from build123d import *

# Parameters (mm, degrees)
ESQUISSE1_W             = 40
ESQUISSE1_H             = 35
ESQUISSE1_W_2           = 36
ESQUISSE1_H_2           = 31
BOSS_EXTRU_1_DEPTH      = 5.5
ESQUISSE2_W             = 40
ESQUISSE2_H             = 35
BOSS_EXTRU_2_DEPTH      = 2
ENL_V_MAT_EXTRU_1_REACH = 42
BOSS_EXTRU_3_DEPTH      = 7
ENL_V_MAT_EXTRU_2_REACH = 11
ESQUISSE9_W             = 7.5
ESQUISSE9_H             = 12
D_GAGEMENT_M31_D        = 3.4
CONG_1_R                = 2.5
BOSS_EXTRU_6_DEPTH      = 1.5


with BuildPart() as part:
    # Esquisse1 → Boss.-Extru.1 (new body)
    with BuildSketch(Plane.XY):
        with Locations((16.877269095, -24.858015503)):
            Rectangle(ESQUISSE1_W, ESQUISSE1_H)
        with Locations((16.877269095, -24.858015503)):
            Rectangle(ESQUISSE1_W_2, ESQUISSE1_H_2, mode=Mode.SUBTRACT)
    extrude(amount=BOSS_EXTRU_1_DEPTH)

    # Esquisse2 → Boss.-Extru.2 (add)
    with BuildSketch(Plane.XY.offset(5.5)):
        with Locations((16.877269095, -24.858015503)):
            Rectangle(ESQUISSE2_W, ESQUISSE2_H)
    extrude(amount=BOSS_EXTRU_2_DEPTH)

    # Esquisse3 → Enlèv. mat.-Extru.1 (cut, up to next)
    with BuildSketch(Plane(origin=(36.877269095, 0, 0), x_dir=(0, 0, -1), z_dir=(1, 0, 0)), mode=Mode.PRIVATE) as enl_v_mat_extru_1_sk1:
        with BuildLine():
            Line((0, -22.358015503), (0, -27.358015503))
            ThreePointArc((0, -27.358015503), (-2.5, -24.858015503), (0, -22.358015503))
        make_face()
    enl_v_mat_extru_1_tool1 = extrude(enl_v_mat_extru_1_sk1.sketch, amount=-ENL_V_MAT_EXTRU_1_REACH, mode=Mode.PRIVATE) & part.part
    add(enl_v_mat_extru_1_tool1.solids().sort_by_distance((36.877269, -24.858016, 1.061033))[0], mode=Mode.SUBTRACT)

    # Esquisse4 → Boss.-Extru.3 (add)
    with BuildSketch(Plane(origin=(0, 0, 5.5), x_dir=(-1, 0, 0), z_dir=(0, 0, -1))):
        with BuildLine():
            ThreePointArc((-34.877269095, -13.919753195), (-30.579172056, -13.656112542), (-30.315531404, -9.358015503))
            Line((-30.315531404, -9.358015503), (-34.877269095, -9.358015503))
            Line((-34.877269095, -9.358015503), (-34.877269095, -13.919753195))
        make_face()
        with BuildLine():
            Line((-34.877269095, -32.858015503), (-17.877269095, -32.858015503))
            Line((-17.877269095, -32.858015503), (-17.877269095, -40.358015503))
            Line((-17.877269095, -40.358015503), (-15.877269095, -40.358015503))
            Line((-15.877269095, -40.358015503), (-15.877269095, -31.858015503))
            ThreePointArc((-15.877269095, -31.858015503), (-16.170162314, -31.150908722), (-16.877269095, -30.858015503))
            Line((-16.877269095, -30.858015503), (-34.877269095, -30.858015503))
            Line((-34.877269095, -30.858015503), (-34.877269095, -32.858015503))
        make_face()
        with BuildLine():
            Line((-34.877269095, -35.796277812), (-34.877269095, -40.358015503))
            Line((-34.877269095, -40.358015503), (-30.315531404, -40.358015503))
            ThreePointArc((-30.315531404, -40.358015503), (-30.579172056, -36.059918465), (-34.877269095, -35.796277812))
        make_face()
        with BuildLine():
            Line((-17.877269095, -16.858015503), (-34.877269095, -16.858015503))
            Line((-34.877269095, -16.858015503), (-34.877269095, -18.858015503))
            Line((-34.877269095, -18.858015503), (-16.877269095, -18.858015503))
            ThreePointArc((-16.877269095, -18.858015503), (-16.170162314, -18.565122285), (-15.877269095, -17.858015503))
            Line((-15.877269095, -17.858015503), (-15.877269095, -9.358015503))
            Line((-15.877269095, -9.358015503), (-17.877269095, -9.358015503))
            Line((-17.877269095, -9.358015503), (-17.877269095, -16.858015503))
        make_face()
        with BuildLine():
            Line((-3.439006787, -40.358015503), (1.122730905, -40.358015503))
            Line((1.122730905, -40.358015503), (1.122730905, -35.796277812))
            ThreePointArc((1.122730905, -35.796277812), (-3.175366134, -36.059918465), (-3.439006787, -40.358015503))
        make_face()
        with BuildLine():
            Line((1.122730905, -13.919753195), (1.122730905, -9.358015503))
            Line((1.122730905, -9.358015503), (-3.439006787, -9.358015503))
            ThreePointArc((-3.439006787, -9.358015503), (-3.175366134, -13.656112542), (1.122730905, -13.919753195))
        make_face()
    extrude(amount=BOSS_EXTRU_3_DEPTH)

    # Esquisse9 → Enlèv. mat.-Extru.2 (cut, up to next)
    with BuildSketch(Plane(origin=(6.5, 0, 7.5), x_dir=(-1, 0, 0), z_dir=(0, 0, -1)), mode=Mode.PRIVATE) as enl_v_mat_extru_2_sk1:
        with Locations((-0.377269095, -24.858015503)):
            Rectangle(ESQUISSE9_W, ESQUISSE9_H)
    enl_v_mat_extru_2_tool1 = extrude(enl_v_mat_extru_2_sk1.sketch, amount=ENL_V_MAT_EXTRU_2_REACH, mode=Mode.PRIVATE) & part.part
    add(enl_v_mat_extru_2_tool1.solids().sort_by_distance((6.877269, -24.858016, 7.5))[0], mode=Mode.SUBTRACT)

    # Dégagement M31 (through all)
    with Locations(Plane.XY.offset(7.5)):
        with Locations((0.877269095, -11.358015503), (32.877269095, -38.358015503), (32.877269095, -11.358015503), (0.877269095, -38.358015503)):
            Hole(D_GAGEMENT_M31_D / 2)

    # Congé1
    cong_1_edges = [part.edges().sort_by_distance(p)[0] for p in [
        (-3.122730905, -7.358015503, 3.75),
        (36.877269095, -7.358015503, 3.75),
        (36.877269095, -42.358015503, 3.75),
        (-3.122730905, -42.358015503, 3.75),
    ]]
    fillet(cong_1_edges, radius=CONG_1_R)

    # Esquisse13 → Boss.-Extru.6 (add)
    with BuildSketch(Plane(origin=(0, 0, 0), x_dir=(-1, 0, 0), z_dir=(0, 0, -1))):
        with BuildLine():
            Line((-35.877269095, -27.358015503), (-34.877269095, -27.358015503))
            Line((-34.877269095, -27.358015503), (-34.877269095, -39.858015503))
            ThreePointArc((-34.877269095, -39.858015503), (-34.730822486, -40.211568894), (-34.377269095, -40.358015503))
            Line((-34.377269095, -40.358015503), (0.622730905, -40.358015503))
            ThreePointArc((0.622730905, -40.358015503), (0.976284295, -40.211568894), (1.122730905, -39.858015503))
            Line((1.122730905, -39.858015503), (1.122730905, -9.861767147))
            ThreePointArc((1.122730905, -9.861767147), (0.975185464, -9.505560944), (0.618979261, -9.358015503))
            Line((0.618979261, -9.358015503), (-34.377269095, -9.358015503))
            ThreePointArc((-34.377269095, -9.358015503), (-34.730822486, -9.504462113), (-34.877269095, -9.858015503))
            Line((-34.877269095, -9.858015503), (-34.877269095, -22.358015503))
            Line((-34.877269095, -22.358015503), (-35.877269095, -22.358015503))
            Line((-35.877269095, -22.358015503), (-35.877269095, -9.858015503))
            ThreePointArc((-35.877269095, -9.858015503), (-35.437929267, -8.797355332), (-34.377269095, -8.358015503))
            Line((-34.377269095, -8.358015503), (0.622730905, -8.358015503))
            ThreePointArc((0.622730905, -8.358015503), (1.683391077, -8.797355332), (2.122730905, -9.858015503))
            Line((2.122730905, -9.858015503), (2.122730905, -39.858015503))
            ThreePointArc((2.122730905, -39.858015503), (1.683391077, -40.918675675), (0.622730905, -41.358015503))
            Line((0.622730905, -41.358015503), (-34.377269095, -41.358015503))
            ThreePointArc((-34.377269095, -41.358015503), (-35.437929267, -40.918675675), (-35.877269095, -39.858015503))
            Line((-35.877269095, -39.858015503), (-35.877269095, -27.358015503))
        make_face()
    extrude(amount=BOSS_EXTRU_6_DEPTH)


solid = part.part
For this review, take the finished solid that the model builds, in its own axes (mm). A direction names the side the tool comes from. Give positions to 0.01 mm unless a question says otherwise; leave off trailing zeros. Loops run counter-clockwise (first coordinate to the right, second up) from the corner with the lowest first, then second, coordinate; pieces in that order, holes last. Notation, with made-up numbers: (2.5, 68) -> (45.5, 68) arc R15 cw to (45.5, 90) -> close; hole circle Ø8 at (-5, 2). An arc over 180 degrees is marked (long way). One line per question, with ' | ' between items.
1) For faces 1 (the flat face through (17, -8.358, -1)), 2 (the flat face through (7, -18.858, 7)), 3 (the flat face through (35.4, -27.358, -0.7)), 4 (the cylindrical face through (16.178, -18.573, 2.049)), list the 3-axis set-ups (+Z, -Z, +X, -X, +Y, -Y) from which the entire face can be reached by the end or side of a thin tool; tool diameter is ignored.
Resolved:
face 1: -Z, +X, -X, +Y | face 2: +Z, -Z | face 3: -Z, +X | face 4: -Z
2) To check wall thickness, follow probe 1 along Y at (x, z) = (22.5, 1.75); probe 2 along Y at (x, z) = (18, -1); probe 3 along X at (y, z) = (-18, 3). State the ranges of each line that lie inside material, in increasing order.
Resolved:
probe 1: y = -42.36 to -40.36, -32.86 to -30.86, -18.86 to -16.86, -9.36 to -7.36 | probe 2: y = -41.36 to -40.36, -32.86 to -30.86, -18.86 to -16.86, -9.36 to -8.36 | probe 3: x = -3.12 to -1.12, 15.89 to 36.88
3) We need section A-A (y = -20.5). Write out the cut boundary in (x, z), plus the area to 3 significant figures.
Resolved:
outline: (-3.12, 0) -> (-2.12, 0) -> (-2.12, -1.5) -> (-1.12, -1.5) -> (-1.12, 5.5) -> (3.13, 5.5) -> (3.13, 7.5) -> (-3.12, 7.5) -> close; (10.63, 5.5) -> (34.88, 5.5) -> (34.88, -1.5) -> (35.88, -1.5) -> (35.88, 0) -> (36.88, 0) -> (36.88, 7.5) -> (10.63, 7.5) -> close | area: 90.0 mm2
4) We need section D-D (y = -25). Write out the cut boundary in (x, z).
Resolved:
outline: (-3.12, 0) -> (-2.12, 0) -> (-2.12, -1.5) -> (-1.12, -1.5) -> (-1.12, 5.5) -> (3.13, 5.5) -> (3.13, 7.5) -> (-3.12, 7.5) -> close; (10.63, 5.5) -> (34.88, 5.5) -> (34.88, 2.5) -> (36.88, 2.5) -> (36.88, 7.5) -> (10.63, 7.5) -> close
5) The part is to be moulded in two halves that separate along X. For faces 5 (the flat face through (26, -18.858, 2)), 6 (the cylindrical face through (-1.7, -40.9, -0.7)), 7 (the flat face through (17, -41.358, -1)), say which applies: +X half, -X half, draft (parallel to the pull), parting line (faces both ways), or undercut.
Resolved:
face 5: undercut | face 6: -X half | face 7: draft
6) Insertion check: pin 1 Ø2 at (x, y) = (24.5, -13) entering from -Z. The pin has a flat end and moves straight along its axis. Give the tip position at first contact, or say it passes through.
Resolved:
pin 1: stops at z = 5.5
7) We need section C-C (z = 4.75). Give the number of separate pieces and of enclosed holes in the cut face, plus the area to 3 significant figures.
Resolved:
separate pieces: 1 | enclosed holes: 7 | area: 446 mm2
8) We need section B-B (x = 13.5). Write out the cut boundary in (y, z), plus the area to 3 significant figures.
Resolved:
outline: (-42.36, 0) -> (-41.36, 0) -> (-41.36, -1.5) -> (-40.36, -1.5) -> (-40.36, 5.5) -> (-9.36, 5.5) -> (-9.36, -1.5) -> (-8.36, -1.5) -> (-8.36, 0) -> (-7.36, 0) -> (-7.36, 7.5) -> (-42.36, 7.5) -> close | area: 95.0 mm2
